Here's the drawing with two shaded views (mm, measured from the low corner). I have some questions. Give positions to 0.01 mm unless a question says otherwise; leave off trailing zeros. Write each loop counter-clockwise with the first axis right and the second up, starting at its lowest first coordinate (ties: lowest second). Pieces come first, ordered by that corner, then holes. Notation, with made-up numbers: M 48.25,64 L 101.25,64 A8 cw 101.25,73 Z; hole C 57.25,59 d7. An arc over 180 degrees is marked long. Use one line per item in the form item = value.
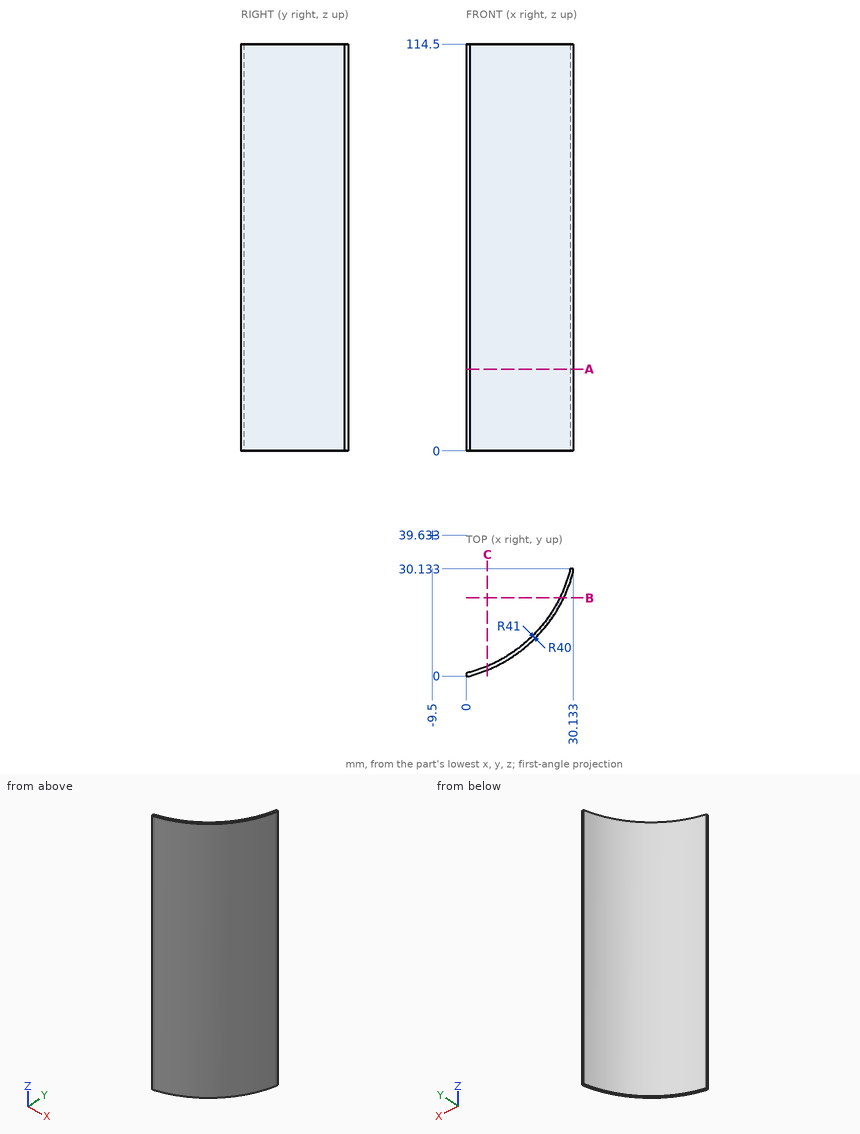
1) I want a section at A-A, the plane z = 23. Please give me the cut outline in (x, y) (1 decimal).
Checked values:
outline = M 0,0 L 1,0 A41 ccw 30.1,29.1 L 30.1,30.1 L 29.4,30.1 A40 cw 0,0.8 Z
2) For pin 1 Ø4 at (x, z) = (5, 15.5) entering from -Y (1 decimal); pin 2 Ø6 at (y, z) = (22, 13.5) entering from -X; pin 3 Ø2 at (y, z) = (10, 53) entering from -X, each with a flat end and sliding along its axis, tell me the tip position at first contact or that it passes through.
Checked values:
pin_1 = 0.6
pin_2 = 24.77
pin_3 = 16.22
3) If I drill on L1, parallel to Y at x = 3, z = 8 (1 decimal); L2, parallel to Y at x = 5.5, z = 87.5 (1 decimal); L3, parallel to X at y = 25, z = 98, over which ranges is the centre line in solid material (lowest first)?
Checked values:
L1 = 0.6 to 1.6
L2 = 1.5 to 2.6
L3 = 27.73 to 28.8
4) I want a section at C-C, the plane x = 6. Please give me the cut outline in (y, z) (1 decimal).
Checked values:
outline = M 1.7,0 L 2.8,0 L 2.8,114.5 L 1.7,114.5 Z
5) I want a section at B-B, the plane y = 22. Please give me the cut outline in (x, z) (1 decimal), plus the area to 3 significant figures.
Checked values:
outline = M 26.4,0 L 27.5,0 L 27.5,114.5 L 26.4,114.5 Z
area = 127 mm2
